Geometry check sheet. Reference: the model listing, model coordinates, mm. A direction names the side the tool comes from. Give positions to 0.01 mm unless a question says otherwise; leave off trailing zeros. Order: outer loops, then holes, each group sorted by start corner. A loop starts at its lowest first (then second) coordinate and runs counter-clockwise, first axis right, second up. Notation, with made-up numbers: M 71.25,-5 L 87.25,-5 A27 cw 87.25,18 Z; hole C 71,65 d11. An arc over 180 degrees is marked long. Answer as CSV lines item,"result". Start each with the question number.
```python
from build123d import *

# Parameters (mm, degrees)
F1_DEPTH = 12
F3_D     = 5
F6_DEPTH = 20.001


with BuildPart() as f1:
    # F0 (on Front) → F1 (new body)
    with BuildSketch(Plane.XZ):
        Polygon((0, 20), (0, 0), (90, 0), (90, 20), (60, 20), (60, 224.426331), (30, 224.426331), (30, 20), align=None)
    extrude(amount=F1_DEPTH)

    # F3 (through all)
    with Locations(Plane.XZ.offset(12)):
        with Locations((38, 212.783181), (38, 176.517542), (38, 147.860397), (38, 113.817503), (38, 74.002333)):
            Hole(F3_D / 2)

    # F4 (on face) + F5 (on face) → F6 (cut, through all)
    with BuildSketch(Plane.XY.offset(20)):
        with BuildLine():
            ThreePointArc((15, -9.3), (12.666548, -8.333452), (11.7, -6))
            ThreePointArc((11.7, -6), (12.666548, -3.666548), (15, -2.7))
            Line((15, -2.7), (7, -2.7))
            ThreePointArc((7, -2.7), (3.7, -6), (7, -9.3))
            Line((7, -9.3), (15, -9.3))
        make_face()
        with BuildLine():
            Line((18.3, -6), (15, -6))
            Line((15, -6), (11.7, -6))
            ThreePointArc((11.7, -6), (12.666548, -8.333452), (15, -9.3))
            ThreePointArc((15, -9.3), (17.333452, -8.333452), (18.3, -6))
        make_face()
        with BuildLine():
            ThreePointArc((15, -2.7), (17.333452, -3.666548), (18.3, -6))
            ThreePointArc((18.3, -6), (17.333452, -8.333452), (15, -9.3))
            Line((15, -9.3), (23, -9.3))
            ThreePointArc((23, -9.3), (26.3, -6), (23, -2.7))
            Line((23, -2.7), (15, -2.7))
        make_face()
        with BuildLine():
            Line((11.7, -6), (15, -6))
            Line((15, -6), (18.3, -6))
            ThreePointArc((18.3, -6), (17.333452, -3.666548), (15, -2.7))
            ThreePointArc((15, -2.7), (12.666548, -3.666548), (11.7, -6))
        make_face()
    with BuildSketch(Plane.XY.offset(20)):
        with BuildLine():
            ThreePointArc((75, -9.3), (72.666548, -8.333452), (71.7, -6))
            ThreePointArc((71.7, -6), (72.666548, -3.666548), (75, -2.7))
            Line((75, -2.7), (67, -2.7))
            ThreePointArc((67, -2.7), (63.7, -6), (67, -9.3))
            Line((67, -9.3), (75, -9.3))
        make_face()
        with BuildLine():
            Line((78.3, -6), (75, -6))
            Line((75, -6), (71.7, -6))
            ThreePointArc((71.7, -6), (72.666548, -8.333452), (75, -9.3))
            ThreePointArc((75, -9.3), (77.333452, -8.333452), (78.3, -6))
        make_face()
        with BuildLine():
            Line((71.7, -6), (75, -6))
            Line((75, -6), (78.3, -6))
            ThreePointArc((78.3, -6), (77.333452, -3.666548), (75, -2.7))
            ThreePointArc((75, -2.7), (72.666548, -3.666548), (71.7, -6))
        make_face()
        with BuildLine():
            ThreePointArc((75, -2.7), (77.333452, -3.666548), (78.3, -6))
            ThreePointArc((78.3, -6), (77.333452, -8.333452), (75, -9.3))
            Line((75, -9.3), (83, -9.3))
            ThreePointArc((83, -9.3), (86.3, -6), (83, -2.7))
            Line((83, -2.7), (75, -2.7))
        make_face()
    extrude(amount=-F6_DEPTH, mode=Mode.SUBTRACT)


solid = f1.part
```
Item 1: Section check B-B on y = -6. Record the boundary of the cut face in (x, z), then the cut area to 3 significant figures.
Item 2: Section check C-C on x = 38. Record the boundary of the cut face in (y, z), then the cut area to 3 significant figures.
Item 3: Depth check by flat-ended pin: pin 1 Ø1.5 at (y, z) = (-2.5, 160) entering from +X; pin 2 Ø1 at (x, y) = (76.5, -9.5) entering from +Z; pin 3 Ø1 at (y, z) = (-10.5, 176) entering from -X. Enter the tip coordinate at first touch or a pass-through.
Item 4: Access from +Z, -Z, +X, -X, +Y, -Y to the whole of each face (thin tool, end or side, straight path). Record for faces 1 (the face through (26.3, -6.1, 10.1)), 2 (the face through (38.33, -5.92, 76.48)), 3 (the face through (15, -2, 20)), 4 (the face through (60, -6, 121)).
Item 5: Scan lines: line 1 along Z through (x, y) = (38, -7.25); line 2 along X through (y, z) = (-6.5, 12); line 3 along Y through (x, z) = (72.5, 12). Record each from-to range of solid material in increasing order.
Item 6: Draft check along Z on faces 5 (the face through (45, -6, 224.426)), 6 (the face through (63.7, -5.9, 10.1)), 7 (the face through (36.66, -5.92, 178.63)). Enter one of: pulls with the +Z half, pulls with the -Z half, needs draft (parallel to the pull), parting line crosses it, or undercut.
Item 7: Section check A-A on x = 72.5. Record the boundary of the cut face in (y, z), then the cut area to 3 significant figures.
Item 8: Section check D-D on z = 133. Record the boundary of the cut face in (x, y), then the cut area to 3 significant figures.
Numbers:
1,outline,"M 0,0 L 3.7,0 L 3.7,20 L 0,20 Z; M 26.3,0 L 63.7,0 L 63.7,20 L 60,20 L 60,224.43 L 30,224.43 L 30,20 L 26.3,20 Z; M 86.3,0 L 90,0 L 90,20 L 86.3,20 Z; hole C 38,74 d5; hole C 38,113.82 d5; hole C 38,147.86 d5; hole C 38,176.52 d5; hole C 38,212.78 d5"
1,area,"6,930 mm2"
2,outline,"M -12,0 L 0,0 L 0,71.5 L -12,71.5 Z; M -12,76.5 L 0,76.5 L 0,111.32 L -12,111.32 Z; M -12,116.32 L 0,116.32 L 0,145.36 L -12,145.36 Z; M -12,150.36 L 0,150.36 L 0,174.02 L -12,174.02 Z; M -12,179.02 L 0,179.02 L 0,210.28 L -12,210.28 Z; M -12,215.28 L 0,215.28 L 0,224.43 L -12,224.43 Z"
2,area,"2,390 mm2"
3,pin 1,"x = 60"
3,pin 2,"z = 20"
3,pin 3,"x = 30"
4,face 1,"+Z, -Z"
4,face 2,"+Y, -Y"
4,face 3,"+Z, -X, +Y, -Y"
4,face 4,"+Z, +X, +Y, -Y"
5,line 1,"0 to 71.5, 76.5 to 111.32, 116.32 to 145.36, 150.36 to 174.02, 179.02 to 210.28, 215.28 to 224.43"
5,line 2,"0 to 3.74, 26.26 to 63.74, 86.26 to 90"
5,line 3,"-12 to -9.3, -2.7 to 0"
6,face 5,"pulls with the +Z half"
6,face 6,"needs draft"
6,face 7,"undercut"
7,outline,"M -12,0 L -9.3,0 L -9.3,20 L -12,20 Z; M -2.7,0 L 0,0 L 0,20 L -2.7,20 Z"
7,area,"108 mm2"
8,outline,"M 30,-12 L 60,-12 L 60,0 L 30,0 Z"
8,area,"360 mm2"
